from build123d import *

# Parameters (mm, degrees)
SKETCH1_R                          = 15
BOSS_EXTRUDE1_DEPTH                = 2
SKETCH2_R                          = 10
BOSS_EXTRUDE2_DEPTH                = 10
SKETCH3_R                          = 4
CUT_EXTRUDE1_DEPTH                 = 25.372115214
SKETCH4_R                          = 1.5
CUT_EXTRUDE2_DEPTH                 = 10
F_3_0_3_DIAMETER_HOLE2_D           = 3
F_3_0_3_DIAMETER_HOLE2_CSINK_D     = 3.05
F_3_0_3_DIAMETER_HOLE2_CSINK_ANGLE = 45


with BuildPart() as part:
    # Sketch1 → Boss-Extrude1 (new body)
    with BuildSketch(Plane(origin=(0, 0, 0), x_dir=(1, 0, 0), z_dir=(0, 1, 0))):
        with Locations(Location((0, 0, 0), (0, 0, 270))):
            Circle(SKETCH1_R)
    extrude(amount=BOSS_EXTRUDE1_DEPTH)

    # Sketch2 → Boss-Extrude2 (add)
    with BuildSketch(Plane(origin=(0, 2, 0), x_dir=(1, 0, 0), z_dir=(0, 1, 0))):
        with Locations(Location((0, 0, 0), (0, 0, 270))):
            Circle(SKETCH2_R)
    extrude(amount=BOSS_EXTRUDE2_DEPTH)

    # Sketch3 → Cut-Extrude1 (cut, through all)
    with BuildSketch(Plane(origin=(0, 12, 0), x_dir=(1, 0, 0), z_dir=(0, 1, 0))):
        with Locations(Location((0, 0, 0), (0, 0, 270))):
            Circle(SKETCH3_R)
    extrude(amount=-CUT_EXTRUDE1_DEPTH, mode=Mode.SUBTRACT)

    # Sketch4 → Cut-Extrude2 (cut)
    with BuildSketch(Plane(origin=(0, 2, 0), x_dir=(1, 0, 0), z_dir=(0, 1, 0))):
        with Locations(Location((-12, 0, 0), (0, 0, 270))):
            Circle(SKETCH4_R)
        with Locations(Location((0, 12, 0), (0, 0, 270))):
            Circle(SKETCH4_R)
        with Locations(Location((12, 0, 0), (0, 0, 270))):
            Circle(SKETCH4_R)
        with Locations(Location((0, -12, 0), (0, 0, 270))):
            Circle(SKETCH4_R)
    extrude(amount=-CUT_EXTRUDE2_DEPTH, mode=Mode.SUBTRACT)

    # Ø3.0 (3) Diameter Hole2 (through all)
    with Locations(Plane(origin=(6.317328185, 6.536355403, 7.751862009), x_dir=(0.775186200902, 0, -0.631732818469), z_dir=(0.631732818469, 0, 0.775186200902))):
        with Locations((0, 0)):
            CounterSinkHole(F_3_0_3_DIAMETER_HOLE2_D / 2, F_3_0_3_DIAMETER_HOLE2_CSINK_D / 2, counter_sink_angle=F_3_0_3_DIAMETER_HOLE2_CSINK_ANGLE)


solid = part.part
CAD build for the part. Positions are in the model's coordinates, mm. A direction names the side the tool comes from. Coordinates: 2 decimals unless noted, no trailing zeros. Write each loop counter-clockwise with the first axis right and the second up, starting at its lowest first coordinate (ties: lowest second). Pieces come first, ordered by that corner, then holes. Notation, with made-up numbers: M -2.75,51.5 L 14.25,51.5 A21 ccw 14.25,77.5 Z; hole C -18,71.25 d7. An arc over 180 degrees is marked long. Answer as a JSON object with one key per item and string values. Group by question number.
1) Saw through at D-D (x = 0.5). Write the cut outline in (y, z).
2) Wall check: line 1 (X direction, y = 0.75, z = 0); line 2 (Y direction, x = -5, z = -11.5); line 3 (X direction, y = 9.25, z = 0). Give the ranges that are in metal, low to high. Write a range as from..to.
3) Saw through at C-C (y = 3). Write the cut outline in (x, z), plus the area to 3 significant figures.
4) Saw through at B-B (z = -12). Write the cut outline in (x, y), plus the area to 3 significant figures.
5) Tool access for faces 1 (the face through (10.2, 2, -0.2)), 2 (the face through (-11.55, 1.01, 1.43)): list every direction of +Z, -Z, +X, -X, +Y, -Y with a clear straight run to the whole face (end or side of a thin tool).
6) Saw through at A-A (x = 12). Write the cut outline in (y, z).
7) Mould opens along X. For faces 3 (the face through (12.45, 1.01, 1.43)), 4 (the face through (0.66, 0.986, -14.985)), 5 (the face through (-3, 0, 3)) say: +X half, -X half, draft (parallel to the pull), parting line (faces both ways), or undercut.
8) Pin check, flat tips, straight feed: pin 1 Ø2.5 at (x, z) = (12, 0) entering from -Y (3 decimals); pin 2 Ø3.5 at (x, z) = (-12, 0) entering from +Y; pin 3 Ø4 at (x, y) = (-7.5, 3) entering from -Z; pin 4 Ø1 at (x, y) = (5.5, 2) entering from -Z. Stop position of each tip, or through.
Values follow:
{
 "1": {"outline": "M 0,-14.99 L 2,-14.99 L 2,-13.41 L 0,-13.41 Z; M 0,-10.59 L 2,-10.59 L 2,-9.99 L 12,-9.99 L 12,-3.97 L 0,-3.97 Z; M 0,3.97 L 12,3.97 L 12,9.99 L 2,9.99 L 2,10.59 L 0,10.59 Z; M 0,13.41 L 2,13.41 L 2,14.99 L 0,14.99 Z"},
 "2": {"line 1": "x = -15..-13.5, -10.5..-4, 4..10.5, 13.5..15", "line 2": "y = 0..2", "line 3": "x = -10..-4, 4..10"},
 "3": {"outline": "C 0,0 d20; hole C 0,0 d8", "area": "264 mm2"},
 "4": {"outline": "M -9,0 L -1.5,0 L -1.5,2 L -9,2 Z; M 1.5,0 L 9,0 L 9,2 L 1.5,2 Z", "area": "30.0 mm2"},
 "5": {"face 1": "+Y", "face 2": "+Y, -Y"},
 "6": {"outline": "M 0,-9 L 2,-9 L 2,-1.5 L 0,-1.5 Z; M 0,1.5 L 2,1.5 L 2,9 L 0,9 Z"},
 "7": {"face 3": "undercut", "face 4": "parting line", "face 5": "draft"},
 "8": {"pin 1": "passes through", "pin 2": "stops at y = 2", "pin 3": "stops at z = -13.85", "pin 4": "stops at z = -14.14"}
}
